Can you work these out from the model? Positions are in its coordinate system, mm. Face numbers are marked on the shaded views. Coordinates: 2 decimals unless noted, no trailing zeros. Loops run counter-clockwise (first coordinate to the right, second up) from the corner with the lowest first, then second, coordinate; pieces in that order, holes last. Notation, with made-up numbers: M 10,55 L 64,55 A18 ccw 64,75 Z; hole C 12.5,32.5 d4. An arc over 180 degrees is marked long. Return JSON: item names as keys, results as strings. Group by question number.
```python
from build123d import *

# Parameters (mm, degrees)
MODEL_R                 = 0.0003
MODEL_R_2               = 0.0002
MODEL_R_3               = 0.00025
MODEL_R_4               = 1.175
MODEL_R_5               = 3.2
MODEL_R_6               = 1.575
SALIENTE_EXTRUIR1_DEPTH = 1.6


with BuildPart() as part:
    # Model → Saliente-Extruir1 (new body)
    # profile 1 of 9: a face of its own
    with BuildSketch(Plane.XY):
        with Locations((-11.66, -6.5)):
            Circle(MODEL_R)
    # profile 2 of 9: a face of its own
    with BuildSketch(Plane.XY):
        with Locations((2.77, -6.5)):
            Circle(MODEL_R)
    # profile 3 of 9: a face of its own
    with BuildSketch(Plane.XY):
        with Locations((9.26, -0.01)):
            Circle(MODEL_R_2)
    # profile 4 of 9: a face of its own
    with BuildSketch(Plane.XY):
        with Locations((9.26, 0.01)):
            Circle(MODEL_R_2)
    # profile 5 of 9: a face of its own
    with BuildSketch(Plane.XY):
        with Locations((2.77, 6.5)):
            Circle(MODEL_R)
    # profile 6 of 9: a face of its own
    with BuildSketch(Plane.XY):
        with Locations((-11.66, 6.5)):
            Circle(MODEL_R)
    # profile 7 of 9: a face of its own
    with BuildSketch(Plane.XY):
        with Locations((-18.15005, 0.01)):
            Circle(MODEL_R_3)
    # profile 8 of 9: a face of its own
    with BuildSketch(Plane.XY):
        with Locations((-18.15005, -0.01)):
            Circle(MODEL_R_3)
    # profile 9 of 9: a face of its own
    with BuildSketch(Plane.XY):
        with BuildLine():
            Line((-11.66, -6.5), (2.77, -6.5))
            ThreePointArc((2.77, -6.5), (7.359079, -4.599079), (9.26, -0.01))
            Line((9.26, -0.01), (9.26, 0.01))
            ThreePointArc((9.26, 0.01), (7.359079, 4.599079), (2.77, 6.5))
            Line((2.77, 6.5), (-11.66, 6.5))
            ThreePointArc((-11.66, 6.5), (-16.249079, 4.599079), (-18.15, 0.01))
            Line((-18.15, 0.01), (-18.15, -0.01))
            ThreePointArc((-18.15, -0.01), (-16.249079, -4.599079), (-11.66, -6.5))
        make_face()
        with Locations((6.2, 0)):
            Circle(MODEL_R_4, mode=Mode.SUBTRACT)
        with Locations((-6.2, 0)):
            Circle(MODEL_R_4, mode=Mode.SUBTRACT)
        Circle(MODEL_R_5, mode=Mode.SUBTRACT)
        with Locations((-12.1, -2)):
            Circle(MODEL_R_6, mode=Mode.SUBTRACT)
    extrude(amount=SALIENTE_EXTRUIR1_DEPTH)


solid = part.part
```
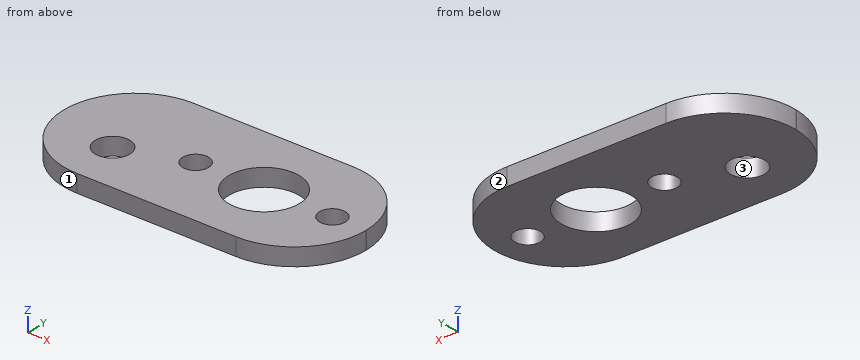
1) Suppose I cut it at D-D, the plane y = -2. List the corners of the cut face in (x, z) for me (3 decimals).
2) If I drill on line 1 (X direction, y = -1, z = 0.7); line 2 (X direction, y = 0.25, z = 0.3); line 3 (Y direction, x = 0, z = 0.7), over which ranges is the centre line in solid material (lowest first)? Write a range as from..to.
3) For pin 1 (4 mm diameter, centred on x = 6.2, y = 0, fed in from -Z); pin 2 (1 mm diameter, centred on x = 1.5, y = 2, fed in from -Z), each with a flat end and sliding along its axis, tell me the tip position at first contact or that it passes through.
4) Suppose I cut it at B-B, the plane x = 0. List the corners of the cut face in (y, z) for me, then the cut area to 3 significant figures.
5) Suppose I cut it at C-C, the plane y = 1.5. List the corners of the cut face in (x, z) for me, then the cut area to 3 significant figures.
6) Suppose I cut it at A-A, the plane z = 1.15. Give the number of separate pieces and of enclosed holes in the cut face, then the cut area to 3 significant figures.
7) If we mould it in two halves opening along X, with no side actions, what happens to the marked faces 1, 2 and 3? For each: +X half, -X half, draft (parallel to the pull), parting line (faces both ways), or undercut.
Returned:
{
 "1": {"outline": "M -17.837,0 L -13.675,0 L -13.675,1.6 L -17.837,1.6 Z; M -10.525,0 L -2.498,0 L -2.498,1.6 L -10.525,1.6 Z; M 2.498,0 L 8.947,0 L 8.947,1.6 L 2.498,1.6 Z"},
 "2": {"line 1": "x = -18.07..-13.32, -10.88..-6.82, -5.58..-3.04, 3.04..5.58, 6.82..9.18", "line 2": "x = -18.15..-7.35, -5.05..-3.19, 3.19..5.05, 7.35..9.26", "line 3": "y = -6.5..-3.2, 3.2..6.5"},
 "3": {"pin 1": "stops at z = 0", "pin 2": "passes through"},
 "4": {"outline": "M -6.5,0 L -3.2,0 L -3.2,1.6 L -6.5,1.6 Z; M 3.2,0 L 6.5,0 L 6.5,1.6 L 3.2,1.6 Z", "area": "10.6 mm²"},
 "5": {"outline": "M -17.98,0 L -2.83,0 L -2.83,1.6 L -17.98,1.6 Z; M 2.83,0 L 9.09,0 L 9.09,1.6 L 2.83,1.6 Z", "area": "34.3 mm²"},
 "6": {"separate pieces": "1", "enclosed holes": "4", "area": "272 mm²"},
 "7": {"face 1": "-X half", "face 2": "+X half", "face 3": "undercut"}
}
